from build123d import *

# Parameters (mm, degrees)
ESQUISSE1_W              = 5
ESQUISSE1_H              = 4.2
ENL_V_MAT_EXTRU_1_DEPTH  = 6
ENL_V_MAT_EXTRU_2_DEPTH  = 6
ENL_V_MAT_EXTRU_3_DEPTH  = 6
ENL_V_MAT_EXTRU_4_DEPTH  = 6
ENL_V_MAT_EXTRU_5_DEPTH  = 6
ENL_V_MAT_EXTRU_6_DEPTH  = 6
ENL_V_MAT_EXTRU_7_DEPTH  = 6
ENL_V_MAT_EXTRU_8_DEPTH  = 6
ENL_V_MAT_EXTRU_9_DEPTH  = 6
ENL_V_MAT_EXTRU_10_DEPTH = 6
ENL_V_MAT_EXTRU_11_DEPTH = 6
ENL_V_MAT_EXTRU_12_DEPTH = 6
ENL_V_MAT_EXTRU_13_DEPTH = 6
ENL_V_MAT_EXTRU_14_DEPTH = 6
ENL_V_MAT_EXTRU_15_DEPTH = 6
ENL_V_MAT_EXTRU_16_DEPTH = 6
ENL_V_MAT_EXTRU_17_DEPTH = 6
ENL_V_MAT_EXTRU_18_DEPTH = 6
ENL_V_MAT_EXTRU_19_DEPTH = 6
ENL_V_MAT_EXTRU_20_DEPTH = 6
ESQUISSE22_W             = 4.14
ESQUISSE22_H             = 2.5
ESQUISSE29_R             = 1.5
ENL_V_MAT_EXTRU_21_DEPTH = 10
BOSS_EXTRU_1_DEPTH       = 9.14


with BuildPart() as part:
    # Esquisse1 → Révolution1 (revolve)
    with BuildSketch(Plane(origin=(0, 0, 0), x_dir=(-1, 0, 0), z_dir=(0, 0, -1))):
        with Locations((0, 2.1)):
            Rectangle(ESQUISSE1_W, ESQUISSE1_H)
    revolve(axis=Axis((2.5, 0, 0), (-1, 0, 0)))

    # Esquisse2 → Enlèv. mat.-Extru.1 (cut, through all)
    with BuildSketch(Plane.ZY.offset(2.5)):
        with BuildLine():
            Line((4.19351351, -0.233333333), (2.714671649, -0.882050288))
            Line((2.714671649, -0.882050288), (3.529773588, -2.276114764))
            ThreePointArc((3.529773588, -2.276114764), (3.994437368, -1.297871376), (4.19351351, -0.233333333))
        make_face()
    extrude(amount=-ENL_V_MAT_EXTRU_1_DEPTH, mode=Mode.SUBTRACT)

    # Esquisse3 → Enlèv. mat.-Extru.2 (cut, through all)
    with BuildSketch(Plane.ZY.offset(2.5)):
        with BuildLine():
            Line((2.557927281, -1.138862601), (3.122928651, -1.58029005))
            Line((3.122928651, -1.58029005), (2.714671649, -0.882050288))
            Line((2.714671649, -0.882050288), (3.455373536, -0.557129899))
            Line((3.455373536, -0.557129899), (2.738813282, -0.582152734))
            ThreePointArc((2.738813282, -0.582152734), (2.662958246, -0.865247584), (2.557927281, -1.138862601))
        make_face()
    extrude(amount=-ENL_V_MAT_EXTRU_2_DEPTH, mode=Mode.SUBTRACT)

    # Esquisse4 → Enlèv. mat.-Extru.3 (cut, through all)
    with BuildSketch(Plane.ZY.offset(2.5)):
        with BuildLine():
            Line((3.255473803, -2.653656028), (1.677759348, -2.309237633))
            Line((1.677759348, -2.309237633), (1.517780128, -3.916164384))
            ThreePointArc((1.517780128, -3.916164384), (2.46869806, -3.397871376), (3.255473803, -2.653656028))
        make_face()
    extrude(amount=-ENL_V_MAT_EXTRU_3_DEPTH, mode=Mode.SUBTRACT)

    # Esquisse5 → Enlèv. mat.-Extru.4 (cut, through all)
    with BuildSketch(Plane.ZY.offset(2.5)):
        with BuildLine():
            Line((1.4, -2.424871131), (1.597631165, -3.114092911))
            Line((1.597631165, -3.114092911), (1.677759348, -2.309237633))
            Line((1.677759348, -2.309237633), (2.467983175, -2.481745162))
            Line((2.467983175, -2.481745162), (1.873565698, -2.080805511))
            ThreePointArc((1.873565698, -2.080805511), (1.645798706, -2.265247584), (1.4, -2.424871131))
        make_face()
    extrude(amount=-ENL_V_MAT_EXTRU_4_DEPTH, mode=Mode.SUBTRACT)

    # Esquisse6 → Enlèv. mat.-Extru.5 (cut, through all)
    with BuildSketch(Plane.ZY.offset(2.5)):
        with BuildLine():
            Line((1.073953753, -4.060372315), (0, -2.85437469))
            Line((0, -2.85437469), (-1.073953753, -4.060372315))
            ThreePointArc((-1.073953753, -4.060372315), (0, -4.2), (1.073953753, -4.060372315))
        make_face()
    extrude(amount=-ENL_V_MAT_EXTRU_5_DEPTH, mode=Mode.SUBTRACT)

    # Esquisse7 → Enlèv. mat.-Extru.6 (cut, through all)
    with BuildSketch(Plane.ZY.offset(2.5)):
        with BuildLine():
            Line((-0.292679697, -2.784661307), (-0.537907124, -3.458418125))
            Line((-0.537907124, -3.458418125), (0, -2.85437469))
            Line((0, -2.85437469), (0.537907124, -3.458418125))
            Line((0.537907124, -3.458418125), (0.292679697, -2.784661307))
            ThreePointArc((0.292679697, -2.784661307), (0, -2.8), (-0.292679697, -2.784661307))
        make_face()
    extrude(amount=-ENL_V_MAT_EXTRU_6_DEPTH, mode=Mode.SUBTRACT)

    # Esquisse8 → Enlèv. mat.-Extru.7 (cut, through all)
    with BuildSketch(Plane.ZY.offset(2.5)):
        with BuildLine():
            Line((-1.517780128, -3.916164384), (-1.677759348, -2.309237633))
            Line((-1.677759348, -2.309237633), (-3.255473803, -2.653656028))
            ThreePointArc((-3.255473803, -2.653656028), (-2.46869806, -3.397871376), (-1.517780128, -3.916164384))
        make_face()
    extrude(amount=-ENL_V_MAT_EXTRU_7_DEPTH, mode=Mode.SUBTRACT)

    # Esquisse9 → Enlèv. mat.-Extru.8 (cut, through all)
    with BuildSketch(Plane.ZY.offset(2.5)):
        with BuildLine():
            Line((-1.873565698, -2.080805511), (-2.467983175, -2.481745162))
            Line((-2.467983175, -2.481745162), (-1.677759348, -2.309237633))
            Line((-1.677759348, -2.309237633), (-1.597631165, -3.114092911))
            Line((-1.597631165, -3.114092911), (-1.4, -2.424871131))
            ThreePointArc((-1.4, -2.424871131), (-1.645798706, -2.265247584), (-1.873565698, -2.080805511))
        make_face()
    extrude(amount=-ENL_V_MAT_EXTRU_8_DEPTH, mode=Mode.SUBTRACT)

    # Esquisse10 → Enlèv. mat.-Extru.9 (cut, through all)
    with BuildSketch(Plane.ZY.offset(2.5)):
        with BuildLine():
            Line((-3.529773588, -2.276114764), (-2.714671649, -0.882050288))
            Line((-2.714671649, -0.882050288), (-4.19351351, -0.233333333))
            ThreePointArc((-4.19351351, -0.233333333), (-3.994437368, -1.297871376), (-3.529773588, -2.276114764))
        make_face()
    extrude(amount=-ENL_V_MAT_EXTRU_9_DEPTH, mode=Mode.SUBTRACT)

    # Esquisse11 → Enlèv. mat.-Extru.10 (cut, through all)
    with BuildSketch(Plane.ZY.offset(2.5)):
        with BuildLine():
            Line((-2.738813282, -0.582152734), (-3.455373536, -0.557129899))
            Line((-3.455373536, -0.557129899), (-2.714671649, -0.882050288))
            Line((-2.714671649, -0.882050288), (-3.122928651, -1.58029005))
            Line((-3.122928651, -1.58029005), (-2.557927281, -1.138862601))
            ThreePointArc((-2.557927281, -1.138862601), (-2.662958246, -0.865247584), (-2.738813282, -0.582152734))
        make_face()
    extrude(amount=-ENL_V_MAT_EXTRU_10_DEPTH, mode=Mode.SUBTRACT)

    # Esquisse12 → Enlèv. mat.-Extru.11 (cut, through all)
    with BuildSketch(Plane.ZY.offset(2.5)):
        with BuildLine():
            Line((-4.19351351, 0.233333333), (-2.714671649, 0.882050288))
            Line((-2.714671649, 0.882050288), (-3.529773588, 2.276114764))
            ThreePointArc((-3.529773588, 2.276114764), (-3.994437368, 1.297871376), (-4.19351351, 0.233333333))
        make_face()
    extrude(amount=-ENL_V_MAT_EXTRU_11_DEPTH, mode=Mode.SUBTRACT)

    # Esquisse13 → Enlèv. mat.-Extru.12 (cut, through all)
    with BuildSketch(Plane.ZY.offset(2.5)):
        with BuildLine():
            Line((-2.714671649, 0.882050288), (-3.455373536, 0.557129899))
            Line((-3.455373536, 0.557129899), (-2.738813282, 0.582152734))
            ThreePointArc((-2.738813282, 0.582152734), (-2.662958246, 0.865247584), (-2.557927281, 1.138862601))
            Line((-2.557927281, 1.138862601), (-3.122928651, 1.58029005))
            Line((-3.122928651, 1.58029005), (-2.714671649, 0.882050288))
        make_face()
    extrude(amount=-ENL_V_MAT_EXTRU_12_DEPTH, mode=Mode.SUBTRACT)

    # Esquisse14 → Enlèv. mat.-Extru.13 (cut, through all)
    with BuildSketch(Plane.ZY.offset(2.5)):
        with BuildLine():
            Line((-3.255473803, 2.653656028), (-1.677759348, 2.309237633))
            Line((-1.677759348, 2.309237633), (-1.517780128, 3.916164384))
            ThreePointArc((-1.517780128, 3.916164384), (-2.46869806, 3.397871376), (-3.255473803, 2.653656028))
        make_face()
    extrude(amount=-ENL_V_MAT_EXTRU_13_DEPTH, mode=Mode.SUBTRACT)

    # Esquisse15 → Enlèv. mat.-Extru.14 (cut, through all)
    with BuildSketch(Plane.ZY.offset(2.5)):
        with BuildLine():
            Line((-1.677759348, 2.309237633), (-2.467983175, 2.481745162))
            Line((-2.467983175, 2.481745162), (-1.873565698, 2.080805511))
            ThreePointArc((-1.873565698, 2.080805511), (-1.645798706, 2.265247584), (-1.4, 2.424871131))
            Line((-1.4, 2.424871131), (-1.597631165, 3.114092911))
            Line((-1.597631165, 3.114092911), (-1.677759348, 2.309237633))
        make_face()
    extrude(amount=-ENL_V_MAT_EXTRU_14_DEPTH, mode=Mode.SUBTRACT)

    # Esquisse16 → Enlèv. mat.-Extru.15 (cut, through all)
    with BuildSketch(Plane.ZY.offset(2.5)):
        with BuildLine():
            Line((-1.073953753, 4.060372315), (0, 2.85437469))
            Line((0, 2.85437469), (1.073953753, 4.060372315))
            ThreePointArc((1.073953753, 4.060372315), (0, 4.2), (-1.073953753, 4.060372315))
        make_face()
    extrude(amount=-ENL_V_MAT_EXTRU_15_DEPTH, mode=Mode.SUBTRACT)

    # Esquisse17 → Enlèv. mat.-Extru.16 (cut, through all)
    with BuildSketch(Plane.ZY.offset(2.5)):
        with BuildLine():
            Line((0, 2.85437469), (-0.537907124, 3.458418125))
            Line((-0.537907124, 3.458418125), (-0.292679697, 2.784661307))
            ThreePointArc((-0.292679697, 2.784661307), (0, 2.8), (0.292679697, 2.784661307))
            Line((0.292679697, 2.784661307), (0.537907124, 3.458418125))
            Line((0.537907124, 3.458418125), (0, 2.85437469))
        make_face()
    extrude(amount=-ENL_V_MAT_EXTRU_16_DEPTH, mode=Mode.SUBTRACT)

    # Esquisse18 → Enlèv. mat.-Extru.17 (cut, through all)
    with BuildSketch(Plane.ZY.offset(2.5)):
        with BuildLine():
            Line((1.517780128, 3.916164384), (1.677759348, 2.309237633))
            Line((1.677759348, 2.309237633), (3.255473803, 2.653656028))
            ThreePointArc((3.255473803, 2.653656028), (2.46869806, 3.397871376), (1.517780128, 3.916164384))
        make_face()
    extrude(amount=-ENL_V_MAT_EXTRU_17_DEPTH, mode=Mode.SUBTRACT)

    # Esquisse19 → Enlèv. mat.-Extru.18 (cut, through all)
    with BuildSketch(Plane.ZY.offset(2.5)):
        with BuildLine():
            Line((1.677759348, 2.309237633), (1.597631165, 3.114092911))
            Line((1.597631165, 3.114092911), (1.4, 2.424871131))
            ThreePointArc((1.4, 2.424871131), (1.645798706, 2.265247584), (1.873565698, 2.080805511))
            Line((1.873565698, 2.080805511), (2.467983175, 2.481745162))
            Line((2.467983175, 2.481745162), (1.677759348, 2.309237633))
        make_face()
    extrude(amount=-ENL_V_MAT_EXTRU_18_DEPTH, mode=Mode.SUBTRACT)

    # Esquisse20 → Enlèv. mat.-Extru.19 (cut, through all)
    with BuildSketch(Plane.ZY.offset(2.5)):
        with BuildLine():
            Line((3.529773588, 2.276114764), (2.714671649, 0.882050288))
            Line((2.714671649, 0.882050288), (4.19351351, 0.233333333))
            ThreePointArc((4.19351351, 0.233333333), (3.994437368, 1.297871376), (3.529773588, 2.276114764))
        make_face()
    extrude(amount=-ENL_V_MAT_EXTRU_19_DEPTH, mode=Mode.SUBTRACT)

    # Esquisse21 → Enlèv. mat.-Extru.20 (cut, through all)
    with BuildSketch(Plane.ZY.offset(2.5)):
        with BuildLine():
            Line((2.714671649, 0.882050288), (3.122928651, 1.58029005))
            Line((3.122928651, 1.58029005), (2.557927281, 1.138862601))
            ThreePointArc((2.557927281, 1.138862601), (2.662958246, 0.865247584), (2.738813282, 0.582152734))
            Line((2.738813282, 0.582152734), (3.455373536, 0.557129899))
            Line((3.455373536, 0.557129899), (2.714671649, 0.882050288))
        make_face()
    extrude(amount=-ENL_V_MAT_EXTRU_20_DEPTH, mode=Mode.SUBTRACT)

    # Esquisse22 → Révolution2 (revolve)
    with BuildSketch(Plane(origin=(0, 0, 0), x_dir=(-1, 0, 0), z_dir=(0, 0, -1))):
        with Locations((-4.57, 1.25)):
            Rectangle(ESQUISSE22_W, ESQUISSE22_H)
    revolve(axis=Axis((6.64, 0, 0), (-1, 0, 0)))

    # Esquisse29 → Enlèv. mat.-Extru.21 (cut)
    with BuildSketch(Plane.ZY.offset(2.5)):
        Circle(ESQUISSE29_R)
    extrude(amount=-ENL_V_MAT_EXTRU_21_DEPTH, mode=Mode.SUBTRACT)

    # Esquisse31 → Boss.-Extru.1 (add)
    with BuildSketch(Plane.ZY.offset(2.5)):
        with BuildLine():
            Line((-0.95, 0), (-0.95, 1.160818677))
            ThreePointArc((-0.95, 1.160818677), (-1.5, 0), (-0.95, -1.160818677))
            Line((-0.95, -1.160818677), (-0.95, 0))
        make_face()
    extrude(amount=-BOSS_EXTRU_1_DEPTH)


solid = part.part
The model under review builds one solid part; all positions refer to its coordinate system, in mm. A direction names the side the tool comes from. Round coordinates to 2 decimals unless told otherwise and drop trailing zeros. Order: outer loops, then holes, each group sorted by start corner. A loop starts at its lowest first (then second) coordinate and runs counter-clockwise, first axis right, second up. Notation, with made-up numbers: (20.5, 6.5) -> (36.5, 6.5) arc R10 cw to (36.5, 15.5) -> close; hole circle Ø3 at (84.25, 71). An arc over 180 degrees is marked (long way). Use CSV: the item, a comma, the result in double quotes. Start each with the question number.
(1) Wall thickness on probe 1 along Z at (x, y) = (0, 0); probe 2 along Y at (x, z) = (1, 0); probe 3 along Y at (x, z) = (4, 0): over which ranges is each line inside the solid? List them lowest first. Write a range as from..to.
(2) Consider section C-C on z = -2.25. Write out the cut boundary in (x, y).
(3) Consider section B-B on z = 0. Write out the cut boundary in (x, y), and give its area (3 significant figures).
(4) Tool access review of faces 4 (the face through (4.54, -0.54, 2.44)), 5 (the face through (-2.5, 0, -2)): name each direction out of +Z, -Z, +X, -X, +Y, -Y from which nothing blocks a thin tool from reaching the whole face with its end or side.
(5) Insertion check: pin 1 (1 mm diameter, centred on x = -0.5, y = 2, fed in from +Z); pin 2 (1.2 mm diameter, centred on x = 4, y = -0.5, fed in from +Z); pin 3 (1 mm diameter, centred on x = -1.5, y = -0.5, fed in from +Z). Each pin has a flat end and moves straight along its axis. Give the tip position at first contact, or say it passes through.
(6) Consider section A-A on y = 0. Write out the cut boundary in (x, z), and give its area (3 significant figures).
(7) Mouldability with a two-part tool opening along Z and no side actions: class faces 1 (the face through (2, 0, -0.95)), 2 (the face through (-0.04, -3.51, 1.56)), 3 (the face through (-0.035, -3.521, -1.557)) as pulls with the +Z half, pulls with the -Z half, needs draft (parallel to the pull), parting line crosses it, or undercut.
Responses:
1,probe 1,"-4.2..-0.95, 1.5..4.2"
1,probe 2,"-2.8..-1.5, 1.5..2.8"
1,probe 3,"-2.5..-1.5, 1.5..2.5"
2,outline,"(-2.5, -2.33) -> (2.5, -2.33) -> (2.5, -1.09) -> (6.64, -1.09) -> (6.64, 1.09) -> (2.5, 1.09) -> (2.5, 2.33) -> (-2.5, 2.33) -> close"
3,outline,"(-2.5, -2.8) -> (2.5, -2.8) -> (2.5, -2.5) -> (6.64, -2.5) -> (6.64, -1.5) -> (-2.5, -1.5) -> close; (-2.5, 1.5) -> (6.64, 1.5) -> (6.64, 2.5) -> (2.5, 2.5) -> (2.5, 2.8) -> (-2.5, 2.8) -> close"
3,area,"21.3 mm²"
4,face 4,"+X"
4,face 5,"+Z, -Z, -X, +Y, -Y"
5,pin 1,"z = 3.53"
5,pin 2,"z = 2.5"
5,pin 3,"z = 4.2"
6,outline,"(-2.5, -4.2) -> (2.5, -4.2) -> (2.5, -2.5) -> (6.64, -2.5) -> (6.64, -0.95) -> (-2.5, -0.95) -> close; (-2.5, 1.5) -> (6.64, 1.5) -> (6.64, 2.5) -> (2.5, 2.5) -> (2.5, 4.2) -> (-2.5, 4.2) -> close"
6,area,"40.3 mm²"
7,face 1,"undercut"
7,face 2,"pulls with the +Z half"
7,face 3,"pulls with the -Z half"
